Can you work these out from the model? Positions are in its coordinate system, mm. Round coordinates to 2 decimals unless told otherwise and drop trailing zeros. Loops run counter-clockwise (first coordinate to the right, second up) from the corner with the lowest first, then second, coordinate; pieces in that order, holes last.
(1) I want a section at A-A on x = -11.69. Write out the boundary of the cut face in (y, z), plus the area to 3 significant figures.
(2) Will this pin go through, and if not, where does the flat tip stop? pin 1 Ø8 at (x, y) = (-11.69, -66.6) entering from +Z.
(3) If I drill on line 1 along Y through (x, z) = (3.81, -1.6); line 2 along X through (y, z) = (-67, -0.8); line 3 along Y through (x, z) = (50, -1.7), over which ranges is the centre line in solid material (lowest first)?
(4) I want a section at B-B on y = -66.6. Write out the boundary of the cut face in (x, z).
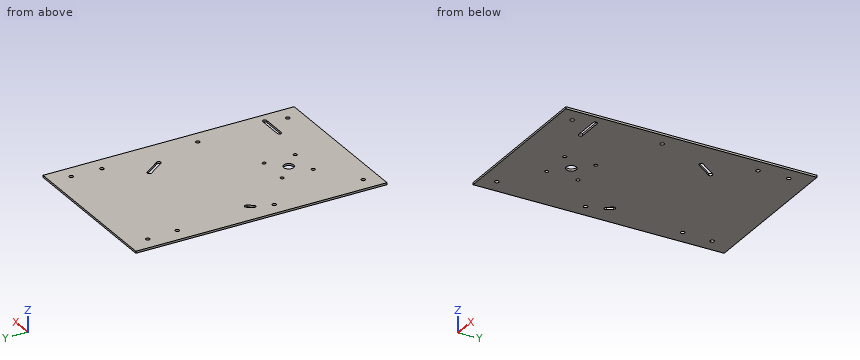
from build123d import *

# Parameters (mm, degrees)
SKETCH1_W           = 160
SKETCH1_H           = 250
BOSS_EXTRUDE1_DEPTH = 2
SKETCH2_R           = 5
SKETCH2_R_2         = 2
CUT_EXTRUDE1_DEPTH  = 149.421696527
SKETCH3_R           = 1.75
CUT_EXTRUDE2_DEPTH  = 10


with BuildPart() as part:
    # Sketch1 → Boss-Extrude1 (new body)
    with BuildSketch(Plane.XY):
        Rectangle(SKETCH1_W, SKETCH1_H)
    extrude(amount=-BOSS_EXTRUDE1_DEPTH)

    # Sketch2 → Cut-Extrude1 (cut, through all)
    with BuildSketch(Plane.XY):
        with Locations((-11.69, -66.6)):
            Circle(SKETCH2_R)
        with Locations((-66, -21)):
            Circle(SKETCH2_R_2)
        with Locations((66, -21)):
            Circle(SKETCH2_R_2)
        with Locations((-66, 105)):
            Circle(SKETCH2_R_2)
        with Locations((66, 105)):
            Circle(SKETCH2_R_2)
        with Locations((65, 75)):
            Circle(SKETCH2_R_2)
        with Locations((-65, 75)):
            Circle(SKETCH2_R_2)
        with Locations((-65, -110)):
            Circle(SKETCH2_R_2)
        with Locations((65, -110)):
            Circle(SKETCH2_R_2)
        with BuildLine():
            Line((70, -92), (45, -92))
            ThreePointArc((45, -92), (43, -90), (45, -88))
            Line((45, -88), (70, -88))
            ThreePointArc((70, -88), (72, -90), (70, -92))
        make_face()
        with BuildLine():
            Line((-54.900342972, 0.015637751), (-58.420342972, -4.843333333))
            ThreePointArc((-58.420342972, -4.843333333), (-61.213333333, -5.289657028), (-61.659657028, -2.496666667))
            Line((-61.659657028, -2.496666667), (-58.139657028, 2.362304418))
            ThreePointArc((-58.139657028, 2.362304418), (-55.346666667, 2.808628113), (-54.900342972, 0.015637751))
        make_face()
        with BuildLine():
            Line((39.928448331, 44.355), (51.678448331, 28.17051669))
            ThreePointArc((51.678448331, 28.17051669), (51.235, 25.377068359), (48.441551669, 25.82051669))
            Line((48.441551669, 25.82051669), (36.691551669, 42.005))
            ThreePointArc((36.691551669, 42.005), (37.135, 44.798448331), (39.928448331, 44.355))
        make_face()
    extrude(amount=-CUT_EXTRUDE1_DEPTH, mode=Mode.SUBTRACT)

    # Sketch3 → Cut-Extrude2 (cut)
    with BuildSketch(Plane.XY):
        with Locations((-27.19, -51.1)):
            Circle(SKETCH3_R)
        with Locations((3.81, -51.1)):
            Circle(SKETCH3_R)
        with Locations((3.81, -82.1)):
            Circle(SKETCH3_R)
        with Locations((-27.19, -82.1)):
            Circle(SKETCH3_R)
    extrude(amount=-CUT_EXTRUDE2_DEPTH, mode=Mode.SUBTRACT)


solid = part.part
Filled sheet:
1. outline: (-125, -2) - (-71.6, -2) - (-71.6, 0) - (-125, 0) - close; (-61.6, -2) - (125, -2) - (125, 0) - (-61.6, 0) - close
1. area: 480 mm2
2. pin 1: passes through
3. line 1: y = -125 to -83.85, -80.35 to -52.85, -49.35 to 125
3. line 2: x = -80 to -16.67, -6.71 to 80
3. line 3: y = -125 to -92, -88 to 25, 30.48 to 125
4. outline: (-80, -2) - (-16.69, -2) - (-16.69, 0) - (-80, 0) - close; (-6.69, -2) - (80, -2) - (80, 0) - (-6.69, 0) - close
